Build history of the part. All positions in model axes, mm. A direction names the side the tool comes from. Round coordinates to 2 decimals unless told otherwise and drop trailing zeros. Order: outer loops, then holes, each group sorted by start corner. A loop starts at its lowest first (then second) coordinate and runs counter-clockwise, first axis right, second up. Notation, with made-up numbers: (-11, -5.5) - (13, -5.5) arc R25 cw to (13, 27.5) - close; hole circle Ø6 at (36, 76.5). An arc over 180 degrees is marked (long way). Write each question's results on one line, items separated by ' | '. Start each with the question number.
Autodesk Inventor part; units mm, degrees
ref_plane "YZ Plane" through (0, 0, 0) normal (1, 0, 0) x (0, 1, 0)
ref_plane "XZ Plane" through (0, 0, 0) normal (0, 1, 0) x (-1, 0, 0)
ref_plane "XY Plane" through (0, 0, 0) normal (0, 0, 1) x (1, 0, 0)
sketch "スケッチ1" plane through (0, 0, 0) normal (0, 0, 1) x (1, 0, 0)
  line L0 (-55, -215) -> (55, -215)
  line L1 (55, -215) -> (55, 215)
  line L2 (55, 215) -> (-55, 215)
  line L3 (-55, 215) -> (-55, -215)
  line L4 (-55, -215) -> (55, 215) construction
  line L5 (55, -215) -> (-55, 215) construction
  line L6 (-55, 185) -> (-50, 185) construction
  line L7 (-50, 185) -> (-25, 210) construction
  line L8 (-25, 210) -> (-25, 215) construction
  line L9 (-46, 95.75) -> (46, 95.75) construction
  line L10 (46, 95.75) -> (46, 187.75) construction
  line L11 (46, 187.75) -> (-46, 187.75) construction
  line L12 (-46, 187.75) -> (-46, 95.75) construction
  line L13 (-46, 95.75) -> (46, 187.75) construction
  line L14 (46, 95.75) -> (-46, 187.75) construction
  line L15 (-46, 1.25) -> (46, 1.25) construction
  line L16 (46, 1.25) -> (46, 93.25) construction
  line L17 (46, 93.25) -> (-46, 93.25) construction
  line L18 (-46, 93.25) -> (-46, 1.25) construction
  line L19 (-46, 1.25) -> (46, 93.25) construction
  line L20 (46, 1.25) -> (-46, 93.25) construction
  line L21 (0, 0) -> (0, 141.75) construction
  circle A0 centre (0, 141.75) radius 53 construction
  line L22 (-44.7, 97.05) -> (44.7, 97.05) construction
  line L23 (44.7, 97.05) -> (44.7, 186.45) construction
  line L24 (44.7, 186.45) -> (-44.7, 186.45) construction
  line L25 (-44.7, 186.45) -> (-44.7, 97.05) construction
  line L26 (-44.7, 97.05) -> (44.7, 186.45) construction
  line L27 (44.7, 97.05) -> (-44.7, 186.45) construction
  arc A1 (-28.4765, 186.45) -> (-44.7, 170.2265) centre (0, 141.75) ccw
  arc A2 (-44.7, 113.2735) -> (-28.4765, 97.05) centre (0, 141.75) ccw
  arc A3 (28.4765, 97.05) -> (44.7, 113.2735) centre (0, 141.75) ccw
  arc A4 (44.7, 170.2265) -> (28.4765, 186.45) centre (0, 141.75) ccw
  line L28 (-28.4765, 186.45) -> (28.4765, 186.45)
  line L29 (-44.7, 170.2265) -> (-44.7, 113.2735)
  line L30 (-28.4765, 97.05) -> (28.4765, 97.05)
  line L31 (44.7, 113.2735) -> (44.7, 170.2265)
  line L32 (-41.25, 100.5) -> (41.25, 100.5) construction
  line L33 (41.25, 100.5) -> (41.25, 183) construction
  line L34 (41.25, 183) -> (-41.25, 183) construction
  line L35 (-41.25, 183) -> (-41.25, 100.5) construction
  line L36 (-41.25, 100.5) -> (41.25, 183) construction
  line L37 (41.25, 100.5) -> (-41.25, 183) construction
  circle A5 centre (-41.25, 183) radius 2.25
  circle A6 centre (-41.25, 100.5) radius 2.25
  circle A7 centre (41.25, 100.5) radius 2.25
  circle A8 centre (41.25, 183) radius 2.25
  circle A9 centre (-41.25, 88.5) radius 2.25
  arc A10 (-28.4765, 91.95) -> (-44.7, 75.7265) centre (0, 47.25) ccw
  line L38 (-28.4765, 91.95) -> (28.4765, 91.95)
  arc A11 (44.7, 75.7265) -> (28.4765, 91.95) centre (0, 47.25) ccw
  circle A12 centre (41.25, 88.5) radius 2.25
  line L39 (44.7, 18.7735) -> (44.7, 75.7265)
  arc A13 (28.4765, 2.55) -> (44.7, 18.7735) centre (0, 47.25) ccw
  circle A14 centre (41.25, 6) radius 2.25
  line L40 (-28.4765, 2.55) -> (28.4765, 2.55)
  circle A15 centre (-41.25, 6) radius 2.25
  arc A16 (-44.7, 18.7735) -> (-28.4765, 2.55) centre (0, 47.25) ccw
  line L41 (-44.7, 75.7265) -> (-44.7, 18.7735)
  circle A17 centre (-41.25, -6) radius 2.25
  arc A18 (-28.4765, -2.55) -> (-44.7, -18.7735) centre (0, -47.25) ccw
  line L42 (-28.4765, -2.55) -> (28.4765, -2.55)
  arc A19 (44.7, -18.7735) -> (28.4765, -2.55) centre (0, -47.25) ccw
  circle A20 centre (41.25, -6) radius 2.25
  line L43 (44.7, -75.7265) -> (44.7, -18.7735)
  arc A21 (28.4765, -91.95) -> (44.7, -75.7265) centre (0, -47.25) ccw
  circle A22 centre (41.25, -88.5) radius 2.25
  line L44 (-28.4765, -91.95) -> (28.4765, -91.95)
  circle A23 centre (-41.25, -88.5) radius 2.25
  arc A24 (-44.7, -75.7265) -> (-28.4765, -91.95) centre (0, -47.25) ccw
  line L45 (-44.7, -18.7735) -> (-44.7, -75.7265)
  circle A25 centre (-41.25, -100.5) radius 2.25
  arc A26 (-28.4765, -97.05) -> (-44.7, -113.2735) centre (0, -141.75) ccw
  line L46 (-28.4765, -97.05) -> (28.4765, -97.05)
  arc A27 (44.7, -113.2735) -> (28.4765, -97.05) centre (0, -141.75) ccw
  circle A28 centre (41.25, -100.5) radius 2.25
  line L47 (44.7, -170.2265) -> (44.7, -113.2735)
  arc A29 (28.4765, -186.45) -> (44.7, -170.2265) centre (0, -141.75) ccw
  circle A30 centre (41.25, -183) radius 2.25
  line L48 (-28.4765, -186.45) -> (28.4765, -186.45)
  circle A31 centre (-41.25, -183) radius 2.25
  arc A32 (-44.7, -170.2265) -> (-28.4765, -186.45) centre (0, -141.75) ccw
  line L49 (-44.7, -113.2735) -> (-44.7, -170.2265)
  circle A33 centre (-45, 205) radius 2.25
  circle A34 centre (45, 205) radius 2.25
  circle A35 centre (45, -205) radius 2.25
  circle A36 centre (-45, -205) radius 2.25
  circle A37 centre (-45, 0) radius 2.25
  circle A38 centre (45, 0) radius 2.25
  line L50 (-55, 0) -> (55, 0) construction
  point P0 (0, 47.25)
  point P1 (0, 47.25)
  dimension "d12" = 106
  dimension "d0" = 110
  dimension "d1" = 430
  dimension "d2" = 135
  dimension "d3" = 30
  dimension "d4" = 30
  dimension "d5" = 5
  dimension "d6" = 92
  dimension "d7" = 92
  dimension "d8" = 92
  dimension "d9" = 92
  dimension "d10" = 2.5
  dimension "d11" = 1.25
  dimension "d13" = 89.4
  dimension "d14" = 89.4
  dimension "d15" = 82.5
  dimension "d16" = 82.5
  dimension "d17" = 4.5
  dimension "d20" = 94.5
  dimension "d25" = 4.5
  dimension "d26" = 10
  dimension "d27" = 10
  dimension "d28" = 10
  dimension "d29" = 10
  dimension "d30" = 10
  dimension "d31" = 10
  dimension "d32" = 10
  dimension "d33" = 10
  dimension "d34" = 10
  dimension "d35" = 10
extrude "押し出し1" add sketch "スケッチ1" along normal blind 3 contours L3 L2 L1 L0 | A37 | A38
sketch "スケッチ2" plane through (0, 0, 3) normal (0, 0, 1) x (1, 0, 0)
  circle A0 centre (-45, 205) radius 2.25 construction
  circle A1 centre (45, -205) radius 2.25 construction
  circle A2 centre (-45, -205) radius 2.25 construction
  circle A3 centre (-43, 203) radius 2.75 construction
  line L0 (55, 215) -> (-55, 215)
  line L1 (-55, 215) -> (-55, -215)
  line L2 (-43.7153, 206.8472) -> (-41.4298, 205.2577)
  line L3 (-45.2577, 201.4298) -> (-46.8472, 203.7153)
  circle A4 centre (-45, 205) radius 2.25 construction
  arc A5 (-43.7153, 206.8472) -> (-46.8472, 203.7153) centre (-45, 205) ccw
  arc A6 (-45.2577, 201.4298) -> (-41.4298, 205.2577) centre (-43, 203) ccw
  line L4 (55, 215) -> (-55, 215) construction
  line L5 (0, 215) -> (0, -215) construction
  line L6 (-55, -215) -> (55, -215) construction
  line L7 (-55, 0) -> (55, 0) construction
  line L8 (55, -215) -> (55, 215) construction
  circle A7 centre (45, 205) radius 2.25 construction
  circle A8 centre (43, 203) radius 2.75 construction
  line L9 (43.7153, 206.8472) -> (41.4298, 205.2577)
  line L10 (45.2577, 201.4298) -> (46.8472, 203.7153)
  circle A9 centre (45, 205) radius 2.25 construction
  arc A10 (46.8472, 203.7153) -> (43.7153, 206.8472) centre (45, 205) ccw
  arc A11 (41.4298, 205.2577) -> (45.2577, 201.4298) centre (43, 203) ccw
  circle A12 centre (-45, -205) radius 2.25 construction
  circle A13 centre (-43, -203) radius 2.75 construction
  line L11 (-43.7153, -206.8472) -> (-41.4298, -205.2577)
  line L12 (-45.2577, -201.4298) -> (-46.8472, -203.7153)
  circle A14 centre (-45, -205) radius 2.25 construction
  arc A15 (-46.8472, -203.7153) -> (-43.7153, -206.8472) centre (-45, -205) ccw
  arc A16 (-41.4298, -205.2577) -> (-45.2577, -201.4298) centre (-43, -203) ccw
  circle A17 centre (45, -205) radius 2.25 construction
  line L13 (45.2577, -201.4298) -> (46.8472, -203.7153)
  arc A18 (45.2577, -201.4298) -> (41.4298, -205.2577) centre (43, -203) ccw
  circle A19 centre (43, -203) radius 2.75 construction
  line L14 (43.7153, -206.8472) -> (41.4298, -205.2577)
  circle A20 centre (45, -205) radius 2.25 construction
  arc A21 (43.7153, -206.8472) -> (46.8472, -203.7153) centre (45, -205) ccw
  point P0 (0, 0)
  dimension "d38" = 5.5
  dimension "d39" = 12
  dimension "d40" = 12
extrude "押し出し2" cut sketch "スケッチ2" against normal through all
sketch "スケッチ4" plane through (0, 0, 3) normal (0, 0, 1) x (1, 0, 0)
  line L0 (55, 215) -> (-55, 215) construction
  line L1 (-28.4765, 186.45) -> (28.4765, 186.45) construction
  line L2 (55, 215) -> (-55, 215) construction
  line L3 (0, 215) -> (0, 186.45) construction
  arc A0 (-17.4739, 209.45) -> (-17.4739, 194.55) centre (-15, 202) ccw construction
  line L4 (-17.4739, 209.45) -> (-12.5261, 209.45) construction
  line L5 (-12.5261, 194.55) -> (-17.4739, 194.55) construction
  arc A1 (-12.5261, 209.45) -> (-17.4739, 209.45) centre (-15, 202) ccw construction
  arc A2 (-12.5261, 194.55) -> (-12.5261, 209.45) centre (-15, 202) ccw construction
  arc A3 (-17.4739, 194.55) -> (-12.5261, 194.55) centre (-15, 202) ccw construction
  line L6 (-17.4755, 194.54) -> (-12.5245, 194.54)
  arc A4 (-12.5245, 194.54) -> (-12.5245, 209.46) centre (-15, 202) ccw
  line L7 (-12.5245, 209.46) -> (-17.4755, 209.46)
  arc A5 (-17.4755, 209.46) -> (-17.4755, 194.54) centre (-15, 202) ccw
  line L8 (-25, 215) -> (-25, 210) construction
  line L9 (-25, 210) -> (-50, 185) construction
  line L10 (-50, 185) -> (-55, 185) construction
  line L11 (-55, 215) -> (-55, -215) construction
  line L12 (17.4755, 194.54) -> (12.5245, 194.54)
  line L13 (12.5245, 209.46) -> (17.4755, 209.46)
  arc A6 (12.5245, 209.46) -> (12.5245, 194.54) centre (15, 202) ccw
  arc A7 (17.4755, 194.54) -> (17.4755, 209.46) centre (15, 202) ccw
  point P0 (0, 0)
  dimension "d46" = 15.7
  dimension "d47" = 14.9
  dimension "d48" = 0.01
  dimension "d49" = 13
  dimension "d50" = 15
  dimension "d51" = 135
  dimension "d52" = 30
  dimension "d53" = 5
extrude "押し出し4" cut sketch "スケッチ4" against normal through all
sketch "スケッチ3" plane through (0, 0, 0) normal (0, 0, -1) x (-1, 0, 0)
  line L0 (-55, 215) -> (55, 215) construction
  line L1 (-55, -215) -> (-55, 215) construction
  line L2 (55, -215) -> (-55, -215) construction
  line L3 (55, 215) -> (55, -215) construction
  line L4 (54.7, 214.7) -> (-54.7, 214.7)
  line L5 (-54.7, 214.7) -> (-54.7, -214.7)
  line L6 (-54.7, -214.7) -> (54.7, -214.7)
  line L7 (54.7, -214.7) -> (54.7, 214.7)
  point P0 (0, 0)
  dimension "d43" = 0.3
extrude "押し出し3" cut sketch "スケッチ3" against normal through all keep common part
equation "\"d4\" = d3"
equation "\"d11\" = 0.5 * d10"
equation "\"d20\" = d7 + d10"
equation "\"d27\" = d26"
equation "\"d28\" = d26"
equation "\"d29\" = d26"
equation "\"d30\" = d26"
equation "\"d31\" = d26"
equation "\"d32\" = d26"
equation "\"d33\" = d26"
equation "\"d34\" = d26"
equation "\"d35\" = d26"
properties part number "front_panel_2" material "アルミニウム 6061"
1. Cut at C-C (x = -32.5). List the corners of the cut face in (y, z).
2. Cut at D-D (z = 1.6). Give the number of separate pieces and of enclosed holes in the cut face, plus the area to 3 significant figures.
3. Mould opens along Y. For faces 1 (the face through (-37.362, -179.341, 1.479)), 2 (the face through (-37, 3, 0)), 3 (the face through (37.362, 179.341, 1.479)) say: pulls with the +Y half, pulls with the -Y half, needs draft (parallel to the pull), parting line crosses it, or undercut.
4. Wall check: line 1 (Y direction, x = -30, z = 0.45); line 2 (X direction, y = -35, z = 0.6); line 3 (Y direction, x = 22, z = 1.9). Give the ranges that are in metal, low to high. Write a range as from..to.
5. Cut at A-A (x = -3). List the corners of the cut face in (y, z).
6. Cut at B-B (y = 148.5). List the corners of the cut face in (x, z).
7. 3-axis set-ups, long thin cutter, end or side, ignore diameter. For faces 4 (the face through (-37.362, -84.841, 1.479)), 5 (the face through (-37, 3, 3)): which of +Z, -Z, +X, -X, +Y, -Y reach the whole face in a straight line?
A:
1) outline: (-214.7, 0) - (-183.62, 0) - (-183.62, 3) - (-214.7, 3) - close; (-99.88, 0) - (-89.12, 0) - (-89.12, 3) - (-99.88, 3) - close; (-5.38, 0) - (5.38, 0) - (5.38, 3) - (-5.38, 3) - close; (89.12, 0) - (99.88, 0) - (99.88, 3) - (89.12, 3) - close; (183.62, 0) - (214.7, 0) - (214.7, 3) - (183.62, 3) - close
2) separate pieces: 1 | enclosed holes: 26 | area: 16,000 mm^2
3) face 1: undercut | face 2: needs draft | face 3: undercut
4) line 1: y = -214.7..-185.44, -98.06..-90.94, -3.56..3.56, 90.94..98.06, 185.44..214.7 | line 2: x = -54.7..-44.7, 44.7..54.7 | line 3: y = -214.7..-186.45, -97.05..-91.95, -2.55..2.55, 91.95..97.05, 186.45..198.43, 205.57..214.7
5) outline: (-214.7, 0) - (-186.45, 0) - (-186.45, 3) - (-214.7, 3) - close; (-97.05, 0) - (-91.95, 0) - (-91.95, 3) - (-97.05, 3) - close; (-2.55, 0) - (2.55, 0) - (2.55, 3) - (-2.55, 3) - close; (91.95, 0) - (97.05, 0) - (97.05, 3) - (91.95, 3) - close; (186.45, 0) - (214.7, 0) - (214.7, 3) - (186.45, 3) - close
6) outline: (-54.7, 0) - (-44.7, 0) - (-44.7, 3) - (-54.7, 3) - close; (44.7, 0) - (54.7, 0) - (54.7, 3) - (44.7, 3) - close
7) face 4: +Z, -Z | face 5: +Z, +X, -X, +Y, -Y
